Input: part model. Units: mm. Frame: model coordinates. A direction names the side the tool comes from. Give positions to 0.01 mm unless a question says otherwise; leave off trailing zeros. Write each loop counter-clockwise with the first axis right and the second up, starting at its lowest first coordinate (ties: lowest second). Pieces come first, ordered by that corner, then holes. Notation, with made-up numbers: (49, 4.25) -> (92, 4.25) arc R25 ccw to (92, 27.25) -> close; hole circle Ø10 at (72, 87.25). An arc over 180 degrees is marked (long way). Return JSON: item names as keys, results as strings. Group by question number.
Item 1: Section D-D, the plane x = -53. Return loops of the section in (y, z).
Item 2: Line query: line 1 (Z direction, x = 11, y = 13); line 2 (X direction, y = 7.5, z = 10); line 3 (X direction, y = -7, z = 32). Output: solid intervals per line, ascending. Write a range as [from, to].
Item 3: Section B-B, the plane x = 17. Return loops of the section in (y, z), then the cut area to 3 significant figures.
Item 4: Section C-C, the plane y = 24. Count the separate pieces of the cut face and the enclosed holes in it, then the cut area to 3 significant figures.
Item 5: Pin query (flat end, axial travel): P1, Ø2, axis at x = 52.5, y = 18, coming from the +Z side; P2, Ø6.5, axis at y = 10, z = 17, coming from the -X side; P3, Ø14, axis at y = -14, z = -24, coming from the -X side. Return the tip coordinate at first contact, or that it passes through.
Item 6: Set-up query: faces 4 (the face through (-63, -6.35, -14)), 5 (the face through (91, -6.35, -14)), 6 (the face through (-6.651, 9, 129)), 7 (the face through (70, 4, 21.225)), 8 (the face through (-19.326, 9, -13)). Return all of +Z, -Z, +X, -X, +Y, -Y with unobstructed straight access to the full face (end or side cutting, diameter ignored); none if empty.
Item 7: Section A-A, the plane z = 27. Return loops of the section in (x, y), then the cut area to 3 significant figures.
Item 8: Mould query, pull axis Y, two halves, no side actions, for faces 1 (the face through (40.339, 9, 59)), 2 (the face through (14, -6.35, 129)), 3 (the face through (13, 6.35, 129)). Classes: released by +Y, released by -Y, zero draft, split by the parting line, or undercut.
from build123d import *

# Parameters (mm, degrees)
BOSS_EXTRUDE1_DEPTH  = 26.9875
BOSS_EXTRUDE5_START  = -6.35
BOSS_EXTRUDE5_DEPTH  = 6.35
SKETCH3_W            = 36.83
SKETCH3_H            = 33.3375
BOSS_EXTRUDE7_DEPTH  = 96.52
SKETCH6_W            = 20.32
SKETCH6_H            = 33.3375
BOSS_EXTRUDE8_DEPTH  = 22.86
SKETCH7_W            = 22.86
SKETCH7_H            = 14.5415
SKETCH7_H_2          = 6.604
CUT_EXTRUDE1_DEPTH   = 21.082
SKETCH11_W           = 39.850701562
SKETCH11_H           = 7.9375
CUT_EXTRUDE3_DEPTH   = 13.716
SHELL1_START         = 3.81
SHELL1_DEPTH         = 23.1775
SHELL1_START_2       = 25.4635
SHELL1_2_DEPTH       = 1.524
SKETCH16_W           = 73.66
SKETCH16_H           = 166.37
BOSS_EXTRUDE9_DEPTH  = 12.7
CUT_EXTRUDE6_START   = -12.7
CUT_EXTRUDE6_DEPTH   = 12.7
SKETCH13_R           = 1.2446
CUT_EXTRUDE4_DEPTH   = 50.8
SKETCH20_W           = 61.160461962
SKETCH20_H           = 49.53
CUT_EXTRUDE8_DEPTH   = 35.8775
BOSS_EXTRUDE16_START = -69.85
SKETCH21_W           = 9.316323924
SKETCH21_H           = 46.0375
SKETCH21_W_2         = 9.316323925
BOSS_EXTRUDE16_DEPTH = 69.85
SKETCH22_W           = 22.86
SKETCH22_H           = 14.5415
SKETCH22_H_2         = 6.604
CUT_EXTRUDE9_DEPTH   = 19.558
SKETCH23_R           = 3.81
CUT_EXTRUDE10_DEPTH  = 36.068


# Read off the part's stored shape, not the designer's step: Shell1
with BuildPart() as part:
    # Sketch1 → Boss-Extrude1 (new body)
    with BuildSketch(Plane(origin=(0, 0, 0), x_dir=(1, 0, 0), z_dir=(0, 1, 0))):
        with BuildLine():
            ThreePointArc((-27.606252307, 13.699523808), (-37.835547974, 38.395228141), (-62.531252307, 48.624523808))
            Line((-62.531252307, 48.624523808), (-62.531252307, 45.513023808))
            ThreePointArc((-62.531252307, 45.513023808), (-40.035710723, 36.195065391), (-30.717752307, 13.699523808))
            ThreePointArc((-30.717752307, 13.699523808), (-40.035710723, -8.796017775), (-62.531252307, -18.113976192))
            Line((-62.531252307, -18.113976192), (-62.531252307, -21.225476192))
            ThreePointArc((-62.531252307, -21.225476192), (-37.835547974, -10.996180525), (-27.606252307, 13.699523808))
        make_face()
        with BuildLine():
            Line((-62.531252307, 45.513023808), (-62.531252307, 48.624523808))
            ThreePointArc((-62.531252307, 48.624523808), (-68.595914912, 48.093934582), (-74.476305812, 46.518288589))
            Line((-74.476305812, 46.518288589), (-73.412110136, 43.594434999))
            ThreePointArc((-73.412110136, 43.594434999), (-68.055608607, 45.029705258), (-62.531252307, 45.513023808))
        make_face()
        with BuildLine():
            ThreePointArc((-74.476305812, -19.119240973), (-68.595914912, -20.694886966), (-62.531252307, -21.225476192))
            Line((-62.531252307, -21.225476192), (-62.531252307, -18.113976192))
            ThreePointArc((-62.531252307, -18.113976192), (-68.055608607, -17.630657643), (-73.412110136, -16.195387383))
            Line((-73.412110136, -16.195387383), (-74.476305812, -19.119240973))
        make_face()
        with BuildLine():
            Line((13.668747693, 48.624523808), (-62.531252307, 48.624523808))
            ThreePointArc((-62.531252307, 48.624523808), (-37.835547974, 38.395228141), (-27.606252307, 13.699523808))
            ThreePointArc((-27.606252307, 13.699523808), (-37.835547974, -10.996180525), (-62.531252307, -21.225476192))
            Line((-62.531252307, -21.225476192), (13.668747693, -21.225476192))
            Line((13.668747693, -21.225476192), (13.668747693, 48.624523808))
        make_face()
    boss_extrude1 = extrude(amount=BOSS_EXTRUDE1_DEPTH)

    # Sketch1<5> → Boss-Extrude5 (add)
    with BuildSketch(Plane(origin=(0, 0, 0), x_dir=(1, 0, 0), z_dir=(0, 1, 0)).offset(BOSS_EXTRUDE5_START)):
        with BuildLine():
            Line((-62.531252307, -21.225476192), (13.668747693, -21.225476192))
            Line((13.668747693, -21.225476192), (13.668747693, 48.624523808))
            Line((13.668747693, 48.624523808), (-62.531252307, 48.624523808))
            ThreePointArc((-62.531252307, 48.624523808), (-97.456252307, 13.699523808), (-62.531252307, -21.225476192))
        make_face()
    boss_extrude5 = extrude(amount=BOSS_EXTRUDE5_DEPTH)

    # Mirror1: Boss-Extrude1, Boss-Extrude5 across plane
    add(boss_extrude1.mirror(Plane(origin=(13.668747693, 26.9875, 0), x_dir=(0, 0, 1), z_dir=(1, 0, 0))))
    add(boss_extrude5.mirror(Plane(origin=(13.668747693, 26.9875, 0), x_dir=(0, 0, 1), z_dir=(1, 0, 0))))

    # Sketch3 → Boss-Extrude7 (add)
    with BuildSketch(Plane.XY.offset(21.225476192)):
        with Locations((-4.746252307, 10.31875)):
            Rectangle(SKETCH3_W, SKETCH3_H)
        with Locations((32.083747693, 10.31875)):
            Rectangle(SKETCH3_W, SKETCH3_H)
    extrude(amount=BOSS_EXTRUDE7_DEPTH)

    # Sketch6 → Boss-Extrude8 (add)
    with BuildSketch(Plane.XY.offset(117.745476192)):
        with Locations((3.508747693, 10.31875)):
            Rectangle(SKETCH6_W, SKETCH6_H)
        with Locations((23.828747693, 10.31875)):
            Rectangle(SKETCH6_W, SKETCH6_H)
    extrude(amount=BOSS_EXTRUDE8_DEPTH)

    # Sketch7 → Cut-Extrude1 (cut)
    with BuildSketch(Plane.ZY.offset(6.651252307)):
        with Locations((129.175476192, 19.71675)):
            Rectangle(SKETCH7_W, SKETCH7_H)
        with Locations((129.175476192, 3.048)):
            Rectangle(SKETCH7_W, SKETCH7_H_2)
    extrude(amount=-CUT_EXTRUDE1_DEPTH, mode=Mode.SUBTRACT)

    # Sketch11 → Cut-Extrude3 (cut)
    with BuildSketch(Plane.XY.offset(21.225476192)):
        with Locations((-57.818603088, 11.33475)):
            Rectangle(SKETCH11_W, SKETCH11_H)
    cut_extrude3 = extrude(amount=-CUT_EXTRUDE3_DEPTH, mode=Mode.SUBTRACT)

    # Mirror2: Cut-Extrude3 across plane
    add(cut_extrude3.mirror(Plane.ZY.offset(-13.668747693)), mode=Mode.SUBTRACT)

    # Shell1 outline → Shell1 (cut)
    with BuildSketch(Plane(origin=(0, 0, 0), x_dir=(1, 0, 0), z_dir=(0, 1, 0)).offset(SHELL1_START)):
        with BuildLine():
            Line((-27.733252307, -9.771179169), (-27.733252307, -11.065476192))
            Line((-27.733252307, -11.065476192), (-13.001252307, -11.065476192))
            Line((-13.001252307, -11.065476192), (-13.001252307, -107.585476192))
            Line((-13.001252307, -107.585476192), (40.338747693, -107.585476192))
            Line((40.338747693, -107.585476192), (40.338747693, -11.065476192))
            Line((40.338747693, -11.065476192), (55.070747693, -11.065476192))
            Line((55.070747693, -11.065476192), (55.070747693, -9.771179169))
            ThreePointArc((55.070747693, -9.771179169), (47.902697541, 14.49030625), (55.979671618, 38.464523808))
            Line((55.979671618, 38.464523808), (-28.642176231, 38.464523808))
            ThreePointArc((-28.642176231, 38.464523808), (-20.565202155, 14.49030625), (-27.733252307, -9.771179169))
        make_face()
    extrude(amount=SHELL1_DEPTH, mode=Mode.SUBTRACT)

    # Shell1 2 outline → Shell1 2 (cut)
    with BuildSketch(Plane(origin=(0, 0, 0), x_dir=(1, 0, 0), z_dir=(0, 1, 0)).offset(SHELL1_START_2)):
        with BuildLine():
            ThreePointArc((-27.733252307, -9.771179169), (-28.181617576, -10.422609102), (-28.642176231, -11.065476192))
            Line((-28.642176231, -11.065476192), (-27.733252307, -11.065476192))
            Line((-27.733252307, -11.065476192), (-27.733252307, -9.771179169))
        make_face()
        with BuildLine():
            ThreePointArc((55.979671618, -11.065476192), (55.519112962, -10.422609101), (55.070747693, -9.771179169))
            Line((55.070747693, -9.771179169), (55.070747693, -11.065476192))
            Line((55.070747693, -11.065476192), (55.979671618, -11.065476192))
        make_face()
    extrude(amount=SHELL1_2_DEPTH, mode=Mode.SUBTRACT)

    # Sketch16 → Boss-Extrude9 (add)
    with BuildSketch(Plane.XZ.offset(6.35)):
        with Locations((13.668747693, 34.560476192)):
            Rectangle(SKETCH16_W, SKETCH16_H)
    extrude(amount=BOSS_EXTRUDE9_DEPTH)

    # Sketch17 → Cut-Extrude6 (cut)
    with BuildSketch(Plane(origin=(0, 3.81, 0), x_dir=(1, 0, 0), z_dir=(0, 1, 0)).offset(CUT_EXTRUDE6_START)):
        with BuildLine():
            Line((-28.642176231, 38.464523808), (55.979671618, 38.464523808))
            ThreePointArc((55.979671618, 38.464523808), (47.895247693, 13.699523808), (55.979671618, -11.065476192))
            Line((55.979671618, -11.065476192), (40.338747693, -11.065476192))
            Line((40.338747693, -11.065476192), (40.338747693, -107.585476192))
            Line((40.338747693, -107.585476192), (-13.001252307, -107.585476192))
            Line((-13.001252307, -107.585476192), (-13.001252307, -11.065476192))
            Line((-13.001252307, -11.065476192), (-28.642176231, -11.065476192))
            ThreePointArc((-28.642176231, -11.065476192), (-20.557752307, 13.699523808), (-28.642176231, 38.464523808))
        make_face()
    extrude(amount=CUT_EXTRUDE6_DEPTH, mode=Mode.SUBTRACT)

    # Sketch13 → Cut-Extrude4 (cut)
    with BuildSketch(Plane(origin=(0, 26.9875, 0), x_dir=(1, 0, 0), z_dir=(0, 1, 0))):
        with Locations(Location((45.418747693, -16.145476192, 0), (0, 0, 270))):
            Circle(SKETCH13_R)
        with Locations(Location((-18.081252307, -16.145476192, 0), (0, 0, 270))):
            Circle(SKETCH13_R)
        with Locations(Location((-18.081252307, 43.544523808, 0), (0, 0, 270))):
            Circle(SKETCH13_R)
        with Locations(Location((45.418747693, 43.544523808, 0), (0, 0, 270))):
            Circle(SKETCH13_R)
    extrude(amount=-CUT_EXTRUDE4_DEPTH, mode=Mode.SUBTRACT)

    # Sketch20 → Cut-Extrude8 (cut)
    with BuildSketch(Plane(origin=(0, 26.9875, 0), x_dir=(1, 0, 0), z_dir=(0, 1, 0))):
        with Locations((17.578978674, 13.699523808)):
            Rectangle(SKETCH20_W, SKETCH20_H)
    extrude(amount=-CUT_EXTRUDE8_DEPTH, mode=Mode.SUBTRACT)

    # Sketch21 → Boss-Extrude16 (add)
    with BuildSketch(Plane(origin=(0, 0, -48.624523808), x_dir=(-1, 0, 0), z_dir=(0, 0, -1)).offset(BOSS_EXTRUDE16_START)):
        with Locations((23.984014269, 3.96875)):
            Rectangle(SKETCH21_W, SKETCH21_H)
        with Locations((-51.321509656, 3.96875)):
            Rectangle(SKETCH21_W_2, SKETCH21_H)
    extrude(amount=BOSS_EXTRUDE16_DEPTH)

    # Sketch22 → Cut-Extrude9 (cut)
    with BuildSketch(Plane.ZY.offset(-14.430747693)):
        with Locations((129.175476192, 19.71675)):
            Rectangle(SKETCH22_W, SKETCH22_H)
        with Locations((129.175476192, 3.048)):
            Rectangle(SKETCH22_W, SKETCH22_H_2)
    extrude(amount=-CUT_EXTRUDE9_DEPTH, mode=Mode.SUBTRACT)

    # Sketch23 → Cut-Extrude10 (cut)
    with BuildSketch(Plane(origin=(0, 12.446, 0), x_dir=(1, 0, 0), z_dir=(0, 1, 0))):
        with Locations(Location((3.508747693, -129.175476192, 0), (0, 0, 180))):
            Circle(SKETCH23_R)
        with Locations(Location((23.828747693, -129.175476192, 0), (0, 0, 180))):
            Circle(SKETCH23_R)
    extrude(amount=-CUT_EXTRUDE10_DEPTH, mode=Mode.SUBTRACT)


solid = part.part
Answer below:
{
 "1": {"outline": "(-6.35, -48.62) -> (26.99, -48.62) -> (26.99, -44.05) -> (0, -44.05) -> (0, 16.65) -> (7.37, 16.65) -> (7.37, 21.23) -> (-6.35, 21.23) -> close; (15.3, 16.65) -> (26.99, 16.65) -> (26.99, 21.23) -> (15.3, 21.23) -> close"},
 "2": {"line 1": "z = [-48.62, -38.46], [107.59, 117.75]", "line 2": "x = [-37.89, -19.33], [46.66, 65.23]", "line 3": "x = [-23.16, -13], [40.34, 50.5]"},
 "3": {"outline": "(-19.05, -48.62) -> (26.99, -48.62) -> (26.99, -38.46) -> (-8.89, -38.46) -> (-8.89, 107.59) -> (26.99, 107.59) -> (26.99, 117.75) -> (12.45, 117.75) -> (12.45, 140.61) -> (6.35, 140.61) -> (6.35, 117.75) -> (-0.25, 117.75) -> (-0.25, 140.61) -> (-6.35, 140.61) -> (-6.35, 117.75) -> (-19.05, 117.75) -> close", "area": "2,700 mm2"},
 "4": {"separate pieces": "1", "enclosed holes": "5", "area": "6,280 mm2"},
 "5": {"P1": "stops at z = 21.23", "P2": "stops at x = -74.4", "P3": "stops at x = -28.64"},
 "6": {"face 4": "+Z, -Z, -X, -Y", "face 5": "+Z, -Z, +X, -Y", "face 6": "+Z, -X, +Y, -Y", "face 7": "+Z, +X, +Y, -Y", "face 8": "+Y"},
 "7": {"outline": "(-23.16, -19.05) -> (50.5, -19.05) -> (50.5, 26.99) -> (40.34, 26.99) -> (40.34, -8.89) -> (-13, -8.89) -> (-13, 26.99) -> (-23.16, 26.99) -> close", "area": "1,480 mm2"},
 "8": {"face 1": "zero draft", "face 2": "released by -Y", "face 3": "undercut"}
}
